Work out the finished part from the listing and answer in its coordinate system (mm). Round coordinates to 2 decimals unless told otherwise and drop trailing zeros. Order: outer loops, then holes, each group sorted by start corner. A loop starts at its lowest first (then second) coordinate and runs counter-clockwise, first axis right, second up. Notation, with made-up numbers: (32.25, 80.5) -> (45.25, 80.5) arc R14 ccw to (45.25, 106.5) -> close; hole circle Ø8 at (-17.75, -23). An arc over 180 degrees is marked (long way). Use one line per item in the form item = value.
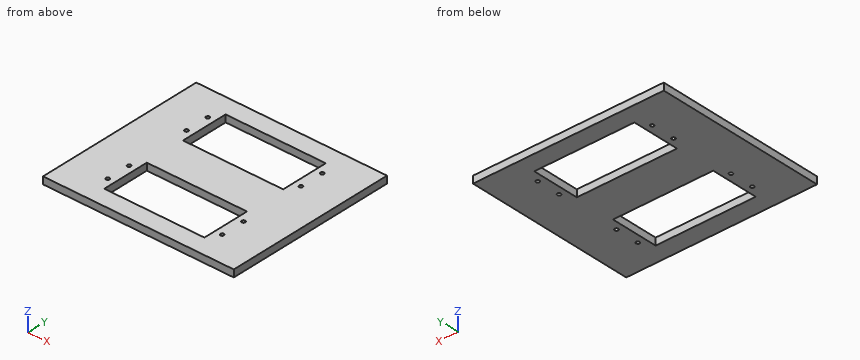
```python
from build123d import *

# Parameters (mm, degrees)
F0_W     = 80
F0_H     = 72
F0_R     = 0.75
F0_W_2   = 42
F0_H_2   = 20
F1_DEPTH = 3


with BuildPart() as f1:
    # F0 (on Top) → F1 (new body)
    with BuildSketch(Plane.XY):
        Rectangle(F0_W, F0_H)
        with Locations((-24, -23.5)):
            Circle(F0_R, mode=Mode.SUBTRACT)
        with Locations((-24, -13.5)):
            Circle(F0_R, mode=Mode.SUBTRACT)
        with Locations((0, -18.5)):
            Rectangle(F0_W_2, F0_H_2, mode=Mode.SUBTRACT)
        with Locations((24, -23.5)):
            Circle(F0_R, mode=Mode.SUBTRACT)
        with Locations((24, -13.5)):
            Circle(F0_R, mode=Mode.SUBTRACT)
        with Locations((-24, 13.5)):
            Circle(F0_R, mode=Mode.SUBTRACT)
        with Locations((-24, 23.5)):
            Circle(F0_R, mode=Mode.SUBTRACT)
        with Locations((24, 13.5)):
            Circle(F0_R, mode=Mode.SUBTRACT)
        with Locations((0, 18.5)):
            Rectangle(F0_W_2, F0_H_2, mode=Mode.SUBTRACT)
        with Locations((24, 23.5)):
            Circle(F0_R, mode=Mode.SUBTRACT)
    extrude(amount=F1_DEPTH)


solid = f1.part
```
Item 1: A flat-ended cylindrical pin translates along its axis: P1, Ø8, axis at x = 9.5, y = -21, coming from the -Z side. Find the tip coordinate at first contact, or state that the pin passes through.
Findings:
P1 = through
Item 2: The part is cut by section B-B, the plane x = 19. Give the vertices of the cut face in (y, z), and give its area (3 significant figures).
Findings:
outline = (-36, 0) -> (-28.5, 0) -> (-28.5, 3) -> (-36, 3) -> close; (-8.5, 0) -> (8.5, 0) -> (8.5, 3) -> (-8.5, 3) -> close; (28.5, 0) -> (36, 0) -> (36, 3) -> (28.5, 3) -> close
area = 96.0 mm^2
Item 3: The part is cut by section C-C, the plane z = 1.7. Give the number of separate pieces and of enclosed holes in the cut face, and give its area (3 significant figures).
Findings:
separate_pieces = 1
enclosed_holes = 10
area = 4,070 mm^2
Item 4: Consider line 1 along Y through (x, z) = (-24, 1.5); line 2 along Y through (x, z) = (-9, 2.85); line 3 along X through (y, z) = (15, 2.25). Determine where each line is inside the solid, lowest interval first.
Findings:
line_1 = -36 to -24.25, -22.75 to -14.25, -12.75 to 12.75, 14.25 to 22.75, 24.25 to 36
line_2 = -36 to -28.5, -8.5 to 8.5, 28.5 to 36
line_3 = -40 to -21, 21 to 40
Item 5: The part is cut by section A-A, the plane y = -15.5. Give the vertices of the cut face in (x, z).
Findings:
outline = (-40, 0) -> (-21, 0) -> (-21, 3) -> (-40, 3) -> close; (21, 0) -> (40, 0) -> (40, 3) -> (21, 3) -> close
